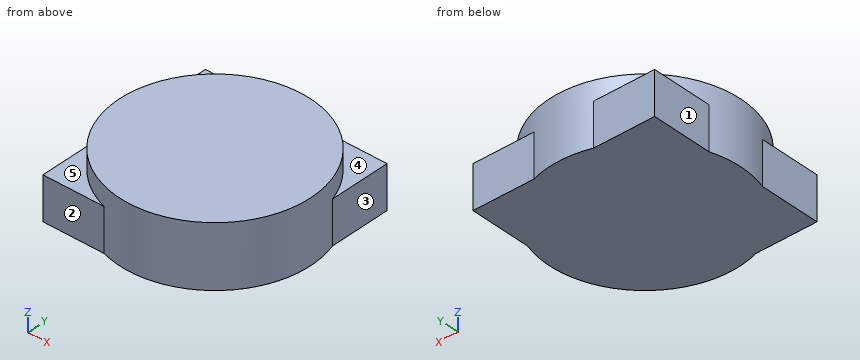
from build123d import *

# Parameters (mm, degrees)
SKETCH1_R           = 20
BOSS_EXTRUDE1_DEPTH = 13
BOSS_EXTRUDE2_DEPTH = 9


with BuildPart() as part:
    # Sketch1 → Boss-Extrude1 (new body)
    with BuildSketch(Plane.XY):
        with Locations(Location((0, 0, 0), (0, 0, 180))):
            Circle(SKETCH1_R)
    extrude(amount=BOSS_EXTRUDE1_DEPTH)

    # Sketch2 → Boss-Extrude2 (add)
    with BuildSketch(Plane(origin=(0, 0, 0), x_dir=(-1, 0, 0), z_dir=(0, 0, -1))):
        with BuildLine():
            Line((-19, 19), (19, 19))
            Line((19, 19), (19, -19))
            Line((19, -19), (-6.244997998, -19))
            ThreePointArc((-6.244997998, -19), (-14.142135624, -14.142135624), (-19, -6.244997998))
            Line((-19, -6.244997998), (-19, 19))
        make_face()
    extrude(amount=-BOSS_EXTRUDE2_DEPTH)


solid = part.part
The listing builds one solid part. Answer for the finished solid, in the listing's coordinates (mm). Face numbers are marked on the shaded views. A direction names the side the tool comes from. Round coordinates to 2 decimals unless told otherwise and drop trailing zeros. Write each loop counter-clockwise with the first axis right and the second up, starting at its lowest first coordinate (ties: lowest second). Pieces come first, ordered by that corner, then holes. Notation, with made-up numbers: M 57.5,46.5 L 91.5,46.5 A8 cw 91.5,58.5 Z; hole C 11,41.25 d10. An arc over 180 degrees is marked long. Write each question's results on one line, items separated by ' | '. Start each with the question number.
Item 1: A cutting plane is placed at B-B on x = -13.5. Write down the section's boundary in (y, z).
Item 2: A cutting plane is placed at C-C on y = 9. Write down the section's boundary in (x, z).
Item 3: Flat-ended cylindrical pins translate along their axes: pin 1 Ø1.5 at (y, z) = (4, 10) entering from +X; pin 2 Ø7 at (y, z) = (-13, 6) entering from -X; pin 3 Ø4.5 at (x, z) = (-11.5, 5.5) entering from +Y. Find the tip coordinate at first contact, or state that the pin passes through.
Item 4: A cutting plane is placed at A-A on z = 6. Write down the section's boundary in (x, y) (3 decimals), and give its area (3 significant figures).
Item 5: Straight lines are drawn through the part: L1, parallel to X at y = 16, z = 3; L2, parallel to X at y = 0.5, z = 9.75. For each, find the intervals that lie inside material, in ascending order. Write a range as [from, to].
Item 6: For the marked faces 1, 2, 3, 4 and 5, determine the directions among +Z, -Z, +X, -X, +Y, -Y from which every point of the face is accessible in a straight line to the end or side of a thin tool.
Item 7: A cutting plane is placed at D-D on x = 11.5. Write down the section's boundary in (y, z), and give its area (3 significant figures).
Check sheet entries:
1) outline: M -19,0 L 19,0 L 19,9 L 14.76,9 L 14.76,13 L -14.76,13 L -14.76,9 L -19,9 Z
2) outline: M -19,0 L 19,0 L 19,9 L 17.86,9 L 17.86,13 L -17.86,13 L -17.86,9 L -19,9 Z
3) pin 1: x = 19.73 | pin 2: x = -19 | pin 3: y = 19
4) outline: M -19,-19 L -6.245,-19 A20 ccw 19,6.245 L 19,19 L 6.245,19 A20 ccw -6.245,19 L -19,19 L -19,6.245 A20 ccw -19,-6.245 Z | area: 1,420 mm²
5) L1: [-19, 19] | L2: [-19.99, 19.99]
6) face 1: +Z, -Z, -X, +Y | face 2: +Z, -Z, -X, -Y | face 3: +Z, -Z, +X, +Y | face 4: +Z, +X, +Y | face 5: +Z, -X, -Y
7) outline: M -16.36,0 L 19,0 L 19,9 L 16.36,9 L 16.36,13 L -16.36,13 Z | area: 449 mm²
